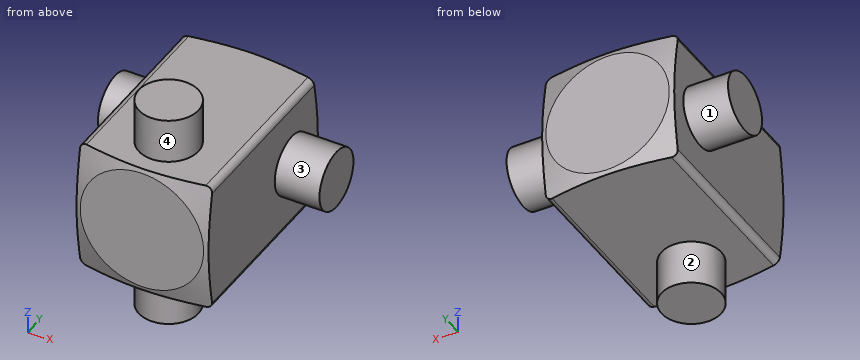
```python
from build123d import *

# Parameters (mm, degrees)
INTERMEDIATE_BODY_SK_W  = 7.874
INTERMEDIATE_BODY_SK_H  = 7.874
INTERMEDIATE_BODY_DEPTH = 11.557
PIN1_R                  = 1.778
PIN_EXTRUDE1_DEPTH      = 6.604
PIN2_R                  = 1.778
PIN_EXTRUDE2_DEPTH      = 6.604
FILLET1_R               = 0.381


with BuildPart() as part:
    # Intermediate_Body-Sk → Intermediate_Body (new body)
    with BuildSketch(Plane(origin=(0, 0, 0), x_dir=(1, 0, 0), z_dir=(0, 1, 0))):
        Rectangle(INTERMEDIATE_BODY_SK_W, INTERMEDIATE_BODY_SK_H)
    extrude(amount=INTERMEDIATE_BODY_DEPTH)

    # Rev-CutSk → Cut-Revolve2 (revolve, cut)
    with BuildSketch(Plane.XY, mode=Mode.PRIVATE) as cut_revolve2_sk:
        Polygon((-3.683, 11.557), (-10.033, 9.855522628), (-10.033, 1.701477372), (-3.683, 0), (-12.573, 0), (-12.573, 11.557), align=None)
    revolve(cut_revolve2_sk.sketch.rotate(Axis((0, 0, 0), (0, 1, 0)), 180), axis=Axis((0, 0, 0), (0, 1, 0)), mode=Mode.SUBTRACT)

    # Pin1 → Pin-Extrude1 (add, symmetric)
    with BuildSketch(Plane.XY):
        with Locations(Location((0, 2.794, 0), (0, 0, 180))):
            Circle(PIN1_R)
    extrude(amount=PIN_EXTRUDE1_DEPTH, both=True)

    # Pin2 → Pin-Extrude2 (add, symmetric)
    with BuildSketch(Plane(origin=(0, 0, 0), x_dir=(0, 0, -1), z_dir=(1, 0, 0))):
        with Locations(Location((0, 8.763, 0), (0, 0, 180))):
            Circle(PIN2_R)
    extrude(amount=PIN_EXTRUDE2_DEPTH, both=True)

    # Fillet1
    fillet1_edges = [part.edges().sort_by_distance(p)[0] for p in [
        (3.937, 5.7785, -3.937),
        (-3.937, 5.7785, -3.937),
        (-3.937, 5.7785, 3.937),
        (3.937, 5.7785, 3.937),
    ]]
    fillet(fillet1_edges, radius=FILLET1_R)


solid = part.part
```
For this review, take the finished solid that the model builds, in its own axes (mm). Face numbers are marked on the shaded views. A direction names the side the tool comes from. Round coordinates to 2 decimals unless told otherwise and drop trailing zeros. Write each loop counter-clockwise with the first axis right and the second up, starting at its lowest first coordinate (ties: lowest second). Pieces come first, ordered by that corner, then holes.
1) Take a section at A-A on x = 0. Give the boundary of the cut face in (y, z).
Answer below:
outline: (0, -3.68) - (0.07, -3.94) - (1.02, -3.94) - (1.02, -6.6) - (4.57, -6.6) - (4.57, -3.94) - (11.49, -3.94) - (11.56, -3.68) - (11.56, 3.68) - (11.49, 3.94) - (4.57, 3.94) - (4.57, 6.6) - (1.02, 6.6) - (1.02, 3.94) - (0.07, 3.94) - (0, 3.68) - close
2) Take a section at C-C on z = 0. Give the boundary of the cut face in (x, y) (3 decimals).
Answer below:
outline: (-6.604, 6.985) - (-3.937, 6.985) - (-3.937, 0.068) - (-3.683, 0) - (3.683, 0) - (3.937, 0.068) - (3.937, 6.985) - (6.604, 6.985) - (6.604, 10.541) - (3.937, 10.541) - (3.937, 11.489) - (3.683, 11.557) - (-3.683, 11.557) - (-3.937, 11.489) - (-3.937, 10.541) - (-6.604, 10.541) - close
3) Take a section at B-B on y = 5.25. Give the boundary of the cut face in (x, z).
Answer below:
outline: (-3.94, -3.56) arc R0.38 ccw to (-3.56, -3.94) - (3.56, -3.94) arc R0.38 ccw to (3.94, -3.56) - (3.94, 3.56) arc R0.38 ccw to (3.56, 3.94) - (-3.56, 3.94) arc R0.38 ccw to (-3.94, 3.56) - close
4) Machinability: for the marked faces 1, 2, 3 and 4, which of the approach directions +Z, -Z, +X, -X, +Y, -Y give a long, thin tool a straight path to every point of the face, cutting with its end or side? Answer none if there is none.
Answer below:
face 1: -X
face 2: -Z
face 3: +X
face 4: +Z
5) Insertion check: pin 1 Ø1.5 at (y, z) = (4.5, 4.5) entering from -X; pin 2 Ø5.5 at (x, y) = (1, 7.5) entering from -Z. Each pin has a flat end and moves straight along its axis. Give the tip position at first contact, or say it passes through.
Answer below:
pin 1: stops at x = -3.88
pin 2: stops at z = -3.94
6) For line 1 along Y through (x, z) = (6.25, 0) (3 decimals); line 2 along Z through (x, y) = (-3.25, 10), list the stretches that pass through material, from the lowest coordinate up.
Answer below:
line 1: y = 6.985 to 10.541
line 2: z = -3.94 to 3.94
7) Take a section at D-D on x = 5.5. Give the boundary of the cut face in (y, z).
Answer below:
outline: circle Ø3.56 at (8.76, 0)
